Geometry check sheet. Reference: the model listing, model coordinates, mm. A direction names the side the tool comes from. Coordinates: 2 decimals unless noted, no trailing zeros. Loops run counter-clockwise (first coordinate to the right, second up) from the corner with the lowest first, then second, coordinate; pieces in that order, holes last. Notation, with made-up numbers: (84.25, -14) - (97.25, -14) arc R14 cw to (97.25, 0) - close; hole circle Ø9 at (-18.75, -36.75). An arc over 180 degrees is marked (long way). One line per item, written item: value.
from build123d import *

# Parameters (mm, degrees)
SKETCH1_W           = 50.8
SKETCH1_H           = 50.8
SKETCH1_R           = 3.175
BOSS_EXTRUDE1_DEPTH = 4.064
SKETCH2_W           = 4.064
SKETCH2_H           = 50.8
BOSS_EXTRUDE2_DEPTH = 50.8
SKETCH3_R           = 15.24
CUT_EXTRUDE1_DEPTH  = 51.8
CUT_EXTRUDE2_DEPTH  = 51.8


with BuildPart() as part:
    # Sketch1 → Boss-Extrude1 (new body)
    with BuildSketch(Plane(origin=(0, 0, 0), x_dir=(1, 0, 0), z_dir=(0, 1, 0))):
        Rectangle(SKETCH1_W, SKETCH1_H)
        Circle(SKETCH1_R, mode=Mode.SUBTRACT)
    extrude(amount=BOSS_EXTRUDE1_DEPTH)

    # Sketch2 → Boss-Extrude2 (add)
    with BuildSketch(Plane(origin=(0, 4.064, 0), x_dir=(1, 0, 0), z_dir=(0, 1, 0))):
        with Locations((-23.368, 0)):
            Rectangle(SKETCH2_W, SKETCH2_H)
        with Locations((23.368, 0)):
            Rectangle(SKETCH2_W, SKETCH2_H)
    extrude(amount=BOSS_EXTRUDE2_DEPTH)

    # Sketch3 → Cut-Extrude1 (cut, through all)
    with BuildSketch(Plane(origin=(25.4, 0, 0), x_dir=(0, 0, -1), z_dir=(1, 0, 0))):
        with Locations((0, 29.464)):
            Circle(SKETCH3_R)
    extrude(amount=-CUT_EXTRUDE1_DEPTH, mode=Mode.SUBTRACT)

    # Sketch4 → Cut-Extrude2 (cut, through all)
    with BuildSketch(Plane.ZY.offset(25.4)):
        with BuildLine():
            ThreePointArc((-25.4, 29.464), (-17.960512262, 47.424512222), (-5.6e-08, 54.864))
            Line((-5.6e-08, 54.864), (-25.4, 54.864))
            Line((-25.4, 54.864), (-25.4, 29.464))
        make_face()
        with BuildLine():
            ThreePointArc((-5.6e-08, 54.864), (17.960512222, 47.424512262), (25.4, 29.464))
            Line((25.4, 29.464), (25.4, 54.864))
            Line((25.4, 54.864), (-5.6e-08, 54.864))
        make_face()
    extrude(amount=-CUT_EXTRUDE2_DEPTH, mode=Mode.SUBTRACT)


solid = part.part
(1) Access from +Z, -Z, +X, -X, +Y, -Y to the whole of each face (thin tool, end or side, straight path). Record for faces 1 (the face through (-0.69, 2, 3.1)), 2 (the face through (-21.336, 18, -11)).
Reply:
face 1: +Y, -Y
face 2: +Z, -Z, +Y
(2) Material ranges on probe 1 along Z at (x, y) = (0, 2.8) (3 decimals); probe 2 along X at (y, z) = (36.5, 18.5); probe 3 along Y at (x, z) = (-22.25, 0), recorded low to high. Write a range as from..to.
Reply:
probe 1: -25.4..-3.175, 3.175..25.4
probe 2: -25.4..-21.34, 21.34..25.4
probe 3: 0..14.22, 44.7..54.86
(3) Cross-section at C-C on z = -2. Record the cut outline in (x, y), and give its area (3 significant figures).
Reply:
outline: (-25.4, 0) - (-2.47, 0) - (-2.47, 4.06) - (-21.34, 4.06) - (-21.34, 14.36) - (-25.4, 14.36) - close; (-25.4, 44.57) - (-21.34, 44.57) - (-21.34, 54.79) - (-25.4, 54.79) - close; (2.47, 0) - (25.4, 0) - (25.4, 14.36) - (21.34, 14.36) - (21.34, 4.06) - (2.47, 4.06) - close; (21.34, 44.57) - (25.4, 44.57) - (25.4, 54.79) - (21.34, 54.79) - close
area: 353 mm2
(4) Cross-section at D-D on y = 31. Record the cut outline in (x, z), and give its area (3 significant figures).
Reply:
outline: (-25.4, -25.35) - (-21.34, -25.35) - (-21.34, -15.16) - (-25.4, -15.16) - close; (-25.4, 15.16) - (-21.34, 15.16) - (-21.34, 25.35) - (-25.4, 25.35) - close; (21.34, -25.35) - (25.4, -25.35) - (25.4, -15.16) - (21.34, -15.16) - close; (21.34, 15.16) - (25.4, 15.16) - (25.4, 25.35) - (21.34, 25.35) - close
area: 166 mm2
(5) Cross-section at B-B on x = 0. Record the cut outline in (y, z) (3 decimals), and give its area (3 significant figures).
Reply:
outline: (0, -25.4) - (4.064, -25.4) - (4.064, -3.175) - (0, -3.175) - close; (0, 3.175) - (4.064, 3.175) - (4.064, 25.4) - (0, 25.4) - close
area: 181 mm2
(6) Cross-section at A-A on y = 7. Record the cut outline in (x, z).
Reply:
outline: (-25.4, -25.4) - (-21.34, -25.4) - (-21.34, 25.4) - (-25.4, 25.4) - close; (21.34, -25.4) - (25.4, -25.4) - (25.4, 25.4) - (21.34, 25.4) - close
(7) Release check for a two-part mould opening along Y. For faces 3 (the face through (4, 4.064, 0)), 4 (the face through (23.396, 44.574, 1.984)), 5 (the face through (-0.1, 3.8, -25.4)), 6 (the face through (5, 0, 0)) record: pulls with the +Y half, pulls with the -Y half, needs draft (parallel to the pull), parting line crosses it, or undercut.
Reply:
face 3: pulls with the +Y half
face 4: undercut
face 5: needs draft
face 6: pulls with the -Y half
(8) Go/stop test with flat-tipped pins: pin 1 Ø1 at (x, z) = (-2, 16) entering from +Y; pin 2 Ø6 at (x, z) = (-1.5, 12) entering from -Y. Record where each tip stops, or that it passes through.
Reply:
pin 1: y = 4.06
pin 2: y = 0
